```python
from build123d import *

# Parameters (mm, degrees)
SKETCH013_W     = 50
SKETCH013_H     = 150
PAD008_DEPTH    = 8
SKETCH014_W     = 50
SKETCH014_H     = 5.4
SKETCH014_H_2   = 101
PAD009_DEPTH    = 10
SKETCH015_R     = 2.75
POCKET003_DEPTH = 18.001
SKETCH016_R     = 3.2
POCKET004_DEPTH = 8
SKETCH017_R     = 15
POCKET005_DEPTH = 18.001
CHAMFER002_SIZE = 1


with BuildPart() as part:
    # Sketch013 → Pad008 (new body)
    with BuildSketch(Plane.XY.offset(-8)):
        Rectangle(SKETCH013_W, SKETCH013_H)
    extrude(amount=PAD008_DEPTH)

    # Sketch014 → Pad009 (join)
    with BuildSketch(Plane.XY):
        with Locations((0, 63)):
            Rectangle(SKETCH014_W, SKETCH014_H)
        with Locations((0, -63)):
            Rectangle(SKETCH014_W, SKETCH014_H)
        Rectangle(SKETCH014_W, SKETCH014_H_2)
    extrude(amount=PAD009_DEPTH)

    # Sketch015 (on Face18 of Pad009) → Pocket003 (cut, through all)
    with BuildSketch(Plane.XY.offset(10)):
        with Locations((-15, 63)):
            Circle(SKETCH015_R)
        with Locations((15, 63)):
            Circle(SKETCH015_R)
        with Locations((-15, -63)):
            Circle(SKETCH015_R)
        with Locations((15, -63)):
            Circle(SKETCH015_R)
    extrude(amount=-POCKET003_DEPTH, mode=Mode.SUBTRACT)

    # Sketch016 (on Face4 of Pocket003) → Pocket004 (cut)
    with BuildSketch(Plane(origin=(0, 0, -8), x_dir=(1, 0, 0), z_dir=(0, 0, -1))):
        with Locations((-15, -63)):
            Circle(SKETCH016_R)
        with Locations((15, -63)):
            Circle(SKETCH016_R)
        with Locations((15, 63)):
            Circle(SKETCH016_R)
        with Locations((-15, 63)):
            Circle(SKETCH016_R)
    extrude(amount=-POCKET004_DEPTH, mode=Mode.SUBTRACT)

    # Sketch017 (on Face26 of Pocket004) → Pocket005 (cut, through all)
    with BuildSketch(Plane.XY.offset(10)):
        Circle(SKETCH017_R)
    extrude(amount=-POCKET005_DEPTH, mode=Mode.SUBTRACT)

    # Chamfer002
    chamfer002_edges = [part.edges().sort_by_distance(p)[0] for p in [
        (-25, 0, 10),
        (0, 50.5, 10),
        (0, -50.5, 10),
        (25, 0, 10),
        (-15, 0, 10),
        (20.261008, 65.7, 10),
        (25, 63, 10),
        (20.261008, 60.3, 10),
        (17.12109, 61.24972, 10),
        (17.12109, 64.75028, 10),
        (0, 65.7, 10),
        (12.25, 63, 10),
        (0, 60.3, 10),
        (-12.87891, 61.24972, 10),
        (-12.87891, 64.75028, 10),
        (-20.261008, 65.7, 10),
        (-17.75, 63, 10),
        (-20.261008, 60.3, 10),
        (-25, 63, 10),
        (20.261008, -60.3, 10),
        (25, -63, 10),
        (20.261008, -65.7, 10),
        (17.12109, -64.75028, 10),
        (17.12109, -61.24972, 10),
        (0, -60.3, 10),
        (12.25, -63, 10),
        (0, -65.7, 10),
        (-12.87891, -64.75028, 10),
        (-12.87891, -61.24972, 10),
        (-20.261008, -60.3, 10),
        (-17.75, -63, 10),
        (-20.261008, -65.7, 10),
        (-25, -63, 10),
        (0, -75, 0),
        (25, -55.4, 0),
        (25, -70.35, 0),
        (-25, -70.35, 0),
        (-25, -55.4, 0),
        (-25, 55.4, 0),
        (25, 55.4, 0),
        (25, 70.35, 0),
        (0, 75, 0),
        (-25, 70.35, 0),
        (-25, 0, -8),
        (0, 75, -8),
        (0, -75, -8),
        (25, 0, -8),
        (-18.2, -63, -8),
        (11.8, -63, -8),
        (-15, 0, -8),
        (-18.2, 63, -8),
        (11.8, 63, -8),
    ]]
    chamfer(chamfer002_edges, length=CHAMFER002_SIZE)


solid = part.part
```
Source: CAD feature listing. Evaluate the final solid. Frame: model axes, mm. A direction names the side the tool comes from. Round coordinates to 2 decimals unless told otherwise and drop trailing zeros. Write each loop counter-clockwise with the first axis right and the second up, starting at its lowest first coordinate (ties: lowest second). Pieces come first, ordered by that corner, then holes. Notation, with made-up numbers: M 2,23.5 L 6,23.5 A5 ccw 6,31.5 Z; hole C 81,11 d1. An arc over 180 degrees is marked long. Answer as a JSON object with one key per item and string values. Group by question number.
(1) Mould query, pull axis Y, two halves, no side actions, for faces 6 (the flat face through (0, -65.7, 4)), 7 (the flat face through (18, 63, 0)), 8 (the conical face through (-12.09, -62.94, 9.16)), 9 (the flat face through (0, 65.7, 4)). Classes: +Y half, -Y half, draft (parallel to the pull), parting line (faces both ways), or undercut.
(2) Section query C-C on y = 0. Output: boundary loops of the cut face in (x, z).
(3) Ray query, line 1 (X direction, y = -63, z = -3.5); line 2 (Y direction, x = 0, z = 1); line 3 (Y direction, x = -20, z = 7.5). Return the intervals inside material, ascending. Write a range as [from, to].
(4) Section query D-D on z = -2.75. Output: boundary loops of the cut face in (x, y).
(5) Reachability of faces 1 (the cylindrical face through (-12.25, -63.05, 4.56)), 2 (the flat face through (25, 16, 1)), 3 (the cylindrical face through (12.461, -61.053, -3.549)), 4 (the conical face through (17.91, 63.06, 9.16)), 5 (the flat face through (0, -60.3, 4)) from +Z, -Z, +X, -X, +Y, -Y: full face, straight path, thin tool, end or side. Return the list, or none.
(6) First-contact query: pin 1 (10 mm diameter, centred on x = 6, z = 6, fed in from +Y); pin 2 (2 mm diameter, centred on x = 17, y = 63.5, fed in from -Z); pin 3 (4.5 mm diameter, centred on x = -22, z = 2.5, fed in from -Y). Flat tips, straight axial feed; report the tip coordinate or a pass-through.
(7) Section query A-A on z = 7. State how many separate pieces and enclosed holes the cut face has, then the cut area to 3 significant figures.
Computed values:
{
 "1": {"face 6": "-Y half", "face 7": "undercut", "face 8": "undercut", "face 9": "+Y half"},
 "2": {"outline": "M -25,-7 L -24,-8 L -16,-8 L -15,-7 L -15,9 L -16,10 L -24,10 L -25,9 Z; M 15,-7 L 16,-8 L 24,-8 L 25,-7 L 25,9 L 24,10 L 16,10 L 15,9 Z"},
 "3": {"line 1": "[-25, -18.2], [-11.8, 11.8], [18.2, 25]", "line 2": "[-65.7, -60.3], [-50.5, -15], [15, 50.5], [60.3, 65.7]", "line 3": "[-65.7, -60.3], [-50.5, 50.5], [60.3, 65.7]"},
 "4": {"outline": "M -25,-75 L 25,-75 L 25,75 L -25,75 Z; hole C -15,-63 d6.4; hole C -15,63 d6.4; hole C 0,0 d30; hole C 15,-63 d6.4; hole C 15,63 d6.4"},
 "5": {"face 1": "+Z, -Z", "face 2": "+Z, -Z, +X, +Y, -Y", "face 3": "-Z", "face 4": "+Z", "face 5": "+Z, +X, -X"},
 "6": {"pin 1": "y = 65.7", "pin 2": "z = 0", "pin 3": "y = -65.7"},
 "7": {"separate pieces": "7", "enclosed holes": "1", "area": "4,790 mm^2"}
}
